from build123d import *

# Parameters (mm, degrees)
BOSS_EXTRUDE1_DEPTH      = 50.8
SKETCH3_W                = 50.8
SKETCH3_H                = 101.6
SKETCH3_R                = 3.175
BOSS_EXTRUDE2_DEPTH      = 3.175
BOSS_EXTRUDE3_DEPTH      = 3.175
BOSS_EXTRUDE3_DEPTH_BACK = 3.175


with BuildPart() as part:
    # Sketch1 → Boss-Extrude1 (new body)
    with BuildSketch(Plane.XY):
        Polygon((0, 0), (12.7, 0), (12.7, 25.4), (9.525, 25.4), (9.525, 3.175), (0, 3.175), align=None)
    extrude(amount=BOSS_EXTRUDE1_DEPTH)

    # Mirror1: part across plane


with BuildPart() as part_1:
    add(part.part)
    add(part.part.mirror(Plane(origin=(0, 3.175, 50.8), x_dir=(0, 0, 1), z_dir=(1, 0, 0))))

    # Sketch3 → Boss-Extrude2 (add)
    with BuildSketch(Plane.ZY.offset(12.7)):
        with Locations((25.4, 12.7)):
            Rectangle(SKETCH3_W, SKETCH3_H)
        with Locations((25.4, 57.15)):
            Circle(SKETCH3_R, mode=Mode.SUBTRACT)
        with Locations((25.4, -31.75)):
            Circle(SKETCH3_R, mode=Mode.SUBTRACT)
    extrude(amount=BOSS_EXTRUDE2_DEPTH)

    # Sketch4 → Boss-Extrude3 (add, two sides: drawn at the far end of the back side and taken through both)
    with BuildSketch(Plane(origin=(0, 0, 25.4), x_dir=(-1, 0, 0), z_dir=(0, 0, -1)).offset(-BOSS_EXTRUDE3_DEPTH_BACK)):
        Polygon((-12.7, 0), (12.7, -25.4), (12.7, 0), align=None)
    extrude(amount=BOSS_EXTRUDE3_DEPTH + BOSS_EXTRUDE3_DEPTH_BACK)


solid = part_1.part
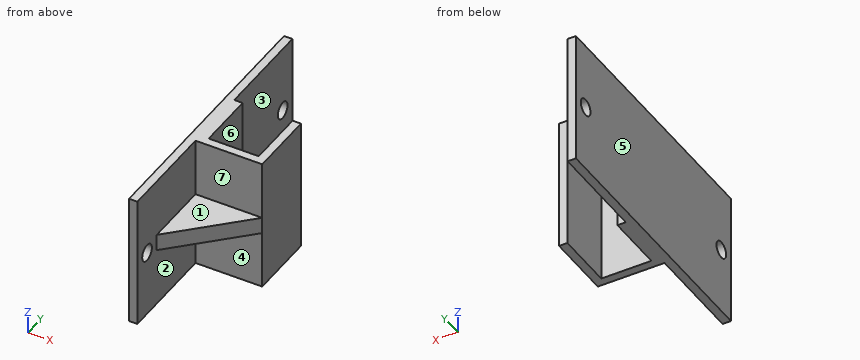
Build history of the part. All positions in model axes, mm. Face numbers are marked on the shaded views. A direction names the side the tool comes from. Round coordinates to 2 decimals unless told otherwise and drop trailing zeros. Write each loop counter-clockwise with the first axis right and the second up, starting at its lowest first coordinate (ties: lowest second). Pieces come first, ordered by that corner, then holes. Notation, with made-up numbers: (-38.75, -2) -> (2.25, -2) arc R35 cw to (2.25, 37) -> close; hole circle Ø5 at (75, -27.75). An arc over 180 degrees is marked (long way). Write item = value, one per line.
(1) Band-saw the part on D-D (z = 8.5). Give the cut face in (x, y) (3 decimals), then the cut area to 3 significant figures.
Answer:
outline = (-15.875, -38.1) -> (-12.7, -38.1) -> (-12.7, 0) -> (12.7, 0) -> (12.7, 25.4) -> (9.525, 25.4) -> (9.525, 3.175) -> (-9.525, 3.175) -> (-9.525, 25.4) -> (-12.7, 25.4) -> (-12.7, 63.5) -> (-15.875, 63.5) -> close
area = 544 mm2
(2) Two-plate mould, pull along X, no slides. Class the marked faces 5, 6 and 7: pulls with the +X half, pulls with the -X half, needs draft (parallel to the pull), parting line crosses it, or undercut.
Answer:
face_5 = pulls with the -X half
face_6 = undercut
face_7 = needs draft
(3) Probe L1, parallel to Y at x = -14.8, z = 25.4 (3 decimals); L2, parallel to X at y = 10.5, z = 5 (3 decimals); L3, parallel to X at y = 49, z = 41 (3 decimals). List the from-to ranges inside material, lowest first.
Answer:
L1 = -38.1 to -34.925, -28.575 to 53.975, 60.325 to 63.5
L2 = -15.875 to -9.525, 9.525 to 12.7
L3 = -15.875 to -12.7
(4) Band-saw the part on A-A (z = 25.4). Give the cut face in (x, y) (3 decimals), then the cut area to 3 significant figures.
Answer:
outline = (-15.875, -38.1) -> (-12.7, -38.1) -> (-12.7, -34.925) -> (-15.875, -34.925) -> close; (-15.875, -28.575) -> (-12.7, -28.575) -> (-12.7, -25.4) -> (12.7, 0) -> (12.7, 25.4) -> (9.525, 25.4) -> (9.525, 3.175) -> (-9.525, 3.175) -> (-9.525, 25.4) -> (-12.7, 25.4) -> (-12.7, 53.975) -> (-15.875, 53.975) -> close; (-15.875, 60.325) -> (-12.7, 60.325) -> (-12.7, 63.5) -> (-15.875, 63.5) -> close
area = 827 mm2
(5) Tool access for the marked faces 1, 2, 3 and 4: list every direction of +Z, -Z, +X, -X, +Y, -Y with a clear straight run to the whole face (end or side of a thin tool).
Answer:
face_1 = +Z, +X, -Y
face_2 = +X, -Y
face_3 = +Z, -Z, +X, +Y
face_4 = -Z, +X, -Y
(6) Band-saw the part on C-C (x = -11.5). Give the cut face in (y, z) (3 decimals).
Answer:
outline = (-24.2, 22.225) -> (0, 22.225) -> (0, 0) -> (25.4, 0) -> (25.4, 50.8) -> (0, 50.8) -> (0, 28.575) -> (-24.2, 28.575) -> close
(7) Flat gauge pins, fed straight in: pin 1 (11 mm diameter, centred on x = 0.5, z = 11.5, fed in from -Y); pin 2 (1 mm diameter, centred on x = -11.5, z = 17.5, fed in from +Y); pin 3 (2 mm diameter, centred on x = -1.5, z = 31.5, fed in from +Y) (3 decimals); pin 4 (7.5 mm diameter, centred on y = 57.15, z = 25.4, fed in from -X) (3 decimals). Where does each tip first touch, or does it go through?
Answer:
pin_1 = 0
pin_2 = 25.4
pin_3 = 3.175
pin_4 = -15.875
(8) Band-saw the part on B-B (y = 5). Give the cut face in (x, z) (3 decimals).
Answer:
outline = (-15.875, 0) -> (-9.525, 0) -> (-9.525, 50.8) -> (-15.875, 50.8) -> close; (9.525, 0) -> (12.7, 0) -> (12.7, 50.8) -> (9.525, 50.8) -> close
